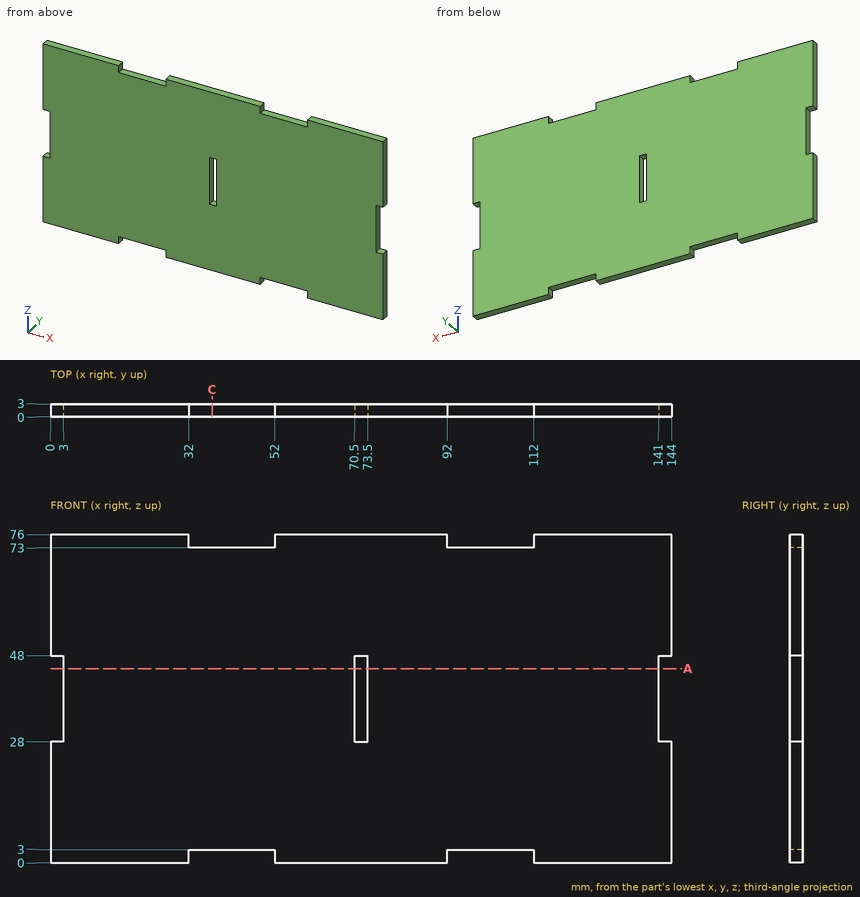
Could you check a few things on this drawing? It's one solid part, dimensions in mm from its lowest x, y, z. Coordinates: 2 decimals unless noted, no trailing zeros. Loops run counter-clockwise (first coordinate to the right, second up) from the corner with the lowest first, then second, coordinate; pieces in that order, holes last. Notation, with made-up numbers: (7.5, 18.5) - (54.5, 18.5) arc R8 cw to (54.5, 30.5) - close; hole circle Ø4 at (33.5, -5). An arc over 180 degrees is marked (long way). Return JSON: item names as keys, results as strings. Group by question number.
Item 1: I need wall thicknesses on line 1 (X direction, y = 2.65, z = 29); line 2 (Z direction, x = 37, y = 2.7). Which ranges of each line are inside material? Lowest first, please. Write a range as from..to.
Item 2: Will these pins go through, and if not, where does the flat tip stop? P1, Ø0.9, axis at x = 42, y = 2, coming from the -Z side; P2, Ø1.5, axis at y = 2.5, z = 31, coming from the +X side.
Item 3: If we section it at A-A on z = 45: Write out the boundary of the cut face in (x, y).
Item 4: If we section it at C-C on x = 37.5: Write out the boundary of the cut face in (y, z), and give its area (3 significant figures).
Calculated:
{
 "1": {"line 1": "x = 3..70.5, 73.5..141", "line 2": "z = 3..73"},
 "2": {"P1": "stops at z = 3", "P2": "stops at x = 141"},
 "3": {"outline": "(3, 0) - (70.5, 0) - (70.5, 3) - (3, 3) - close; (73.5, 0) - (141, 0) - (141, 3) - (73.5, 3) - close"},
 "4": {"outline": "(0, 3) - (3, 3) - (3, 73) - (0, 73) - close", "area": "210 mm^2"}
}
